Input: part model. Units: mm. Frame: model coordinates. A direction names the side the tool comes from. Round coordinates to 2 decimals unless told otherwise and drop trailing zeros. Write each loop counter-clockwise with the first axis right and the second up, starting at its lowest first coordinate (ties: lowest second). Pieces come first, ordered by that corner, then holes. Notation, with made-up numbers: (-7, -18.5) - (16, -18.5) arc R29 ccw to (16, 16.5) - close; hole circle Ø10 at (0.25, -27). An arc over 180 degrees is marked (long way). Use one line per item in the form item = value.
```python
from build123d import *

# Parameters (mm, degrees)
F1_DEPTH       = 11.7
F4_R           = 3
F6_DEPTH       = 0.75
F6_TAPER       = 35
F5_R           = 3
F7_DEPTH       = 0.75
F7_TAPER       = 35
F8_D           = 2.95
F8_CSINK_D     = 5.5
F8_CSINK_ANGLE = 85
F9_D           = 3.3
F9_CBORE_D     = 6.5
F9_CBORE_DEPTH = 4
F10_SIZE       = 1


with BuildPart() as f1:
    # F0 (on Top) → F1 (new body)
    with BuildSketch(Plane.XY):
        Polygon((-13, -7.3), (8, -7.3), (8, 0), (0, 0), (0, -5), (-13, -5), align=None)
        Polygon((0, 0), (8, 0), (8, 7.3), (-13, 7.3), (-13, 5), (0, 5), align=None)
    extrude(amount=F1_DEPTH)

    # F4 (on face) → F6 (join)
    with BuildSketch(Plane(origin=(0, -5, 0), x_dir=(-1, 0, 0), z_dir=(0, 1, 0))):
        with Locations((7.5, 5.85)):
            Circle(F4_R)
    extrude(amount=F6_DEPTH, taper=F6_TAPER)

    # F5 (on face) → F7 (join)
    with BuildSketch(Plane.XZ.offset(-5)):
        with Locations((-7.5, 5.85)):
            Circle(F5_R)
    extrude(amount=F7_DEPTH, taper=F7_TAPER)

    # F8 (through all)
    with Locations(Plane.XZ.offset(7.3)):
        with Locations((-7.5, 5.85)):
            CounterSinkHole(F8_D / 2, F8_CSINK_D / 2, counter_sink_angle=F8_CSINK_ANGLE)

    # F9 (through all)
    with Locations(Plane(origin=(0, 0, 0), x_dir=(0, -1, 0), z_dir=(-1, 0, 0))):
        with Locations((0, 5.85)):
            CounterBoreHole(F9_D / 2, F9_CBORE_D / 2, F9_CBORE_DEPTH)

    # F10
    f10_edges = [f1.edges().sort_by_distance(p)[0] for p in [
        (-13, -6.15, 11.7),
        (-13, -6.15, 0),
        (-13, 6.15, 0),
        (-13, 6.15, 11.7),
        (8, 0, 11.7),
        (8, -7.3, 5.85),
        (8, 0, 0),
        (8, 7.3, 5.85),
    ]]
    chamfer(f10_edges, length=F10_SIZE)


solid = f1.part
```
(1) Material intervals for L1, parallel to Z at x = -7.5, y = 5.65 (3 decimals); L2, parallel to Y at x = -8.25, z = 2.5; L3, parallel to Z at x = 2.7, y = 0, sorted ascending.
Derived:
L1 = 0 to 4.375, 7.325 to 11.7
L2 = -7.3 to -5, 5 to 7.3
L3 = 0 to 2.6, 9.1 to 11.7
(2) Cut plane A-A on y = 0. Output: boundary loops of the cut face in (x, z), then the cut area to 3 significant figures.
Derived:
outline = (0, 0) - (7, 0) - (8, 1) - (8, 4.2) - (4, 4.2) - (4, 2.6) - (0, 2.6) - close; (0, 9.1) - (4, 9.1) - (4, 7.5) - (8, 7.5) - (8, 10.7) - (7, 11.7) - (0, 11.7) - close
area = 53.4 mm^2
(3) First-contact query: pin 1 Ø1.5 at (y, z) = (4, 4) entering from -X; pin 2 Ø2.5 at (y, z) = (0, 5.85) entering from -X; pin 3 Ø1.5 at (x, z) = (-6.5, 5.5) entering from -Y; pin 4 Ø5 at (y, z) = (0, 6) entering from -X. Flat tips, straight axial feed; report the tip coordinate or a pass-through.
Derived:
pin_1 = -9.83
pin_2 = through
pin_3 = -6.27
pin_4 = 4
(4) Draft query along X for faces 4 (the face through (-6.33, 5.8, 4.95)), 5 (the face through (2, 0, 0)), 6 (the face through (8, -1.5, 6.9)). Return one class per face: released by +X, released by -X, zero draft, split by the parting line, or undercut.
Derived:
face_4 = undercut
face_5 = zero draft
face_6 = released by +X
(5) Cut plane C-C on z = 10.25. Output: boundary loops of the cut face in (x, y).
Derived:
outline = (-13, -7.3) - (7, -7.3) - (8, -6.3) - (8, 6.3) - (7, 7.3) - (-13, 7.3) - (-13, 5) - (0, 5) - (0, -5) - (-13, -5) - close
(6) Cut plane B-B on x = 1.25. Output: boundary loops of the cut face in (y, z).
Derived:
outline = (-7.3, 0) - (7.3, 0) - (7.3, 11.7) - (-7.3, 11.7) - close; hole circle Ø6.5 at (0, 5.85)
(7) Cut plane D-D on x = -7.5. Output: boundary loops of the cut face in (y, z) (3 decimals).
Derived:
outline = (-7.3, 0) - (-5, 0) - (-5, 2.85) - (-4.25, 3.375) - (-4.25, 4.375) - (-5.909, 4.375) - (-7.3, 3.1) - close; (-7.3, 8.6) - (-5.909, 7.325) - (-4.25, 7.325) - (-4.25, 8.325) - (-5, 8.85) - (-5, 11.7) - (-7.3, 11.7) - close; (4.25, 3.375) - (5, 2.85) - (5, 0) - (7.3, 0) - (7.3, 4.375) - (4.25, 4.375) - close; (4.25, 7.325) - (7.3, 7.325) - (7.3, 11.7) - (5, 11.7) - (5, 8.85) - (4.25, 8.325) - close
(8) Access query for faces 1 (the face through (-4, -5, 6)), 2 (the face through (-6, 4.25, 5)), 3 (the face through (4, -1, 4)). Directions: +Z, -Z, +X, -X, +Y, -Y. A direction counts if a zero-diameter tool reaches every point of the face in a straight line with its end or side. Return the directions, or none.
Derived:
face_1 = none
face_2 = +Z, -Z, -X
face_3 = -X
